Read the model definition and answer for the solid it produces. Units are mm, in the model's axes. A direction names the side the tool comes from. Coordinates: 2 decimals unless noted, no trailing zeros. Write each loop counter-clockwise with the first axis right and the second up, starting at its lowest first coordinate (ties: lowest second). Pieces come first, ordered by that corner, then holes. Notation, with made-up numbers: (3, -17.75) -> (60, -17.75) arc R32 ccw to (60, 12.25) -> close; hole circle Ø5 at (26.5, 12). An arc over 180 degrees is marked (long way). Answer as a JSON object with one key per item and string values. Group by question number.
(1) Straight lines are drawn through the part: L1, parallel to Z at x = 3.75, y = 32.5; L2, parallel to X at y = 2, z = 2.35; L3, parallel to Y at x = 5.25, z = 1. For each, find the intervals that lie inside material, in ascending order.
(2) Which of the six approach directions +Z, -Z, +X, -X, +Y, -Y give full straight-line access (tool end or side, diameter ignored) to faces 1 (the face through (12.29, 33.33, 2.98)), 2 (the face through (2.958, 0.574, 1.577)), 3 (the face through (6, 2, 1))?
(3) Find section A-A (x = 4.5). Give the vertices of the cut face in (y, z).
(4) For a pull along Y with two mould halves and no side action, classify faces 4 (the face through (1.324, 3.377, 3.342)), 5 (the face through (19, 2, 1)), 6 (the face through (18.886, 3.44, 1.03)) as +Y half, -Y half, draft (parallel to the pull), parting line (faces both ways), or undercut.
(5) Find section B-B (y = 8.5). Give the vertices of the cut face in (x, z).
(6) Find section D-D (z = 3.5). Count the separate pieces of the cut face and the enclosed holes in it, then the cut area to 3 significant figures.
(7) Find section C-C (x = 12.5). Give the vertices of the cut face in (y, z).
(8) Flat-ended cylindrical pins translate along their axes: P1, Ø0.9, axis at y = 2.5, z = 2, coming from the -X side; P2, Ø8, axis at x = 17, y = 22.5, coming from the +Z side. Find the tip coordinate at first contact, or state that the pin passes through.
from build123d import *

# Parameters (mm, degrees)
F2_DEPTH = 25
F4_DEPTH = 3.3107000528
F5_R     = 0.6765328669
F6_DEPTH = 2
F7_R     = 1.6
F8_DEPTH = 3.2


with BuildPart() as f2:
    # F1 (on Right) → F2 (new body)
    with BuildSketch(Plane.YZ):
        Polygon((0, 0), (35, 0), (35, 1.4), (5.8304471904, 1.4), (1.1319840864, 3.1101007166), align=None)
    extrude(amount=F2_DEPTH)

    # F3 (on face) → F4 (cut, through all)
    with BuildSketch(Plane(origin=(0, 1.1319840864, 3.1101007166), x_dir=(1, 0, 0), z_dir=(0, 0.3420201433, 0.9396926208))):
        with BuildLine():
            Line((6, 0), (19, 0))
            Line((19, 0), (19, 2.6))
            ThreePointArc((19, 2.6), (18.8828427125, 2.8828427125), (18.6, 3))
            Line((18.6, 3), (6.4, 3))
            ThreePointArc((6.4, 3), (6.1171572875, 2.8828427125), (6, 2.6))
            Line((6, 2.6), (6, 0))
        make_face()
    extrude(amount=-F4_DEPTH, mode=Mode.SUBTRACT)

    # F5 (on face) → F6 (join)
    with BuildSketch(Plane(origin=(0, 1.1319840864, 3.1101007166), x_dir=(1, 0, 0), z_dir=(0, 0.3420201433, 0.9396926208))):
        with Locations((23, 2)):
            Circle(F5_R)
        with Locations((2, 2)):
            Circle(F5_R)
    extrude(amount=F6_DEPTH)

    # F7 (on face) → F8 (join)
    with BuildSketch(Plane.XY.offset(1.4)):
        with Locations((12.5, 31.7446738482)):
            Circle(F7_R)
    extrude(amount=F8_DEPTH)


solid = f2.part
Results below:
{
 "1": {"L1": "z = 0 to 1.4", "L2": "x = 0 to 6, 19 to 25", "L3": "y = 0.36 to 35"},
 "2": {"face 1": "+Z", "face 2": "+Z, +X, -X, -Y", "face 3": "+Z, -Y"},
 "3": {"outline": "(0, 0) -> (35, 0) -> (35, 1.4) -> (5.83, 1.4) -> (1.13, 3.11) -> close"},
 "4": {"face 4": "undercut", "face 5": "draft", "face 6": "-Y half"},
 "5": {"outline": "(0, 0) -> (25, 0) -> (25, 1.4) -> (0, 1.4) -> close"},
 "6": {"separate pieces": "3", "enclosed holes": "0", "area": "11.1 mm2"},
 "7": {"outline": "(3.19, 0) -> (35, 0) -> (35, 1.4) -> (33.34, 1.4) -> (33.34, 4.6) -> (30.14, 4.6) -> (30.14, 1.4) -> (5.83, 1.4) -> (3.95, 2.08) -> close"},
 "8": {"P1": "stops at x = 0", "P2": "stops at z = 1.4"}
}
